Source: CAD feature listing. Evaluate the final solid. Frame: model axes, mm. Face numbers are marked on the shaded views. A direction names the side the tool comes from. Give positions to 0.01 mm unless a question says otherwise; leave off trailing zeros. Write each loop counter-clockwise with the first axis right and the second up, starting at its lowest first coordinate (ties: lowest second). Pieces come first, ordered by that corner, then holes.
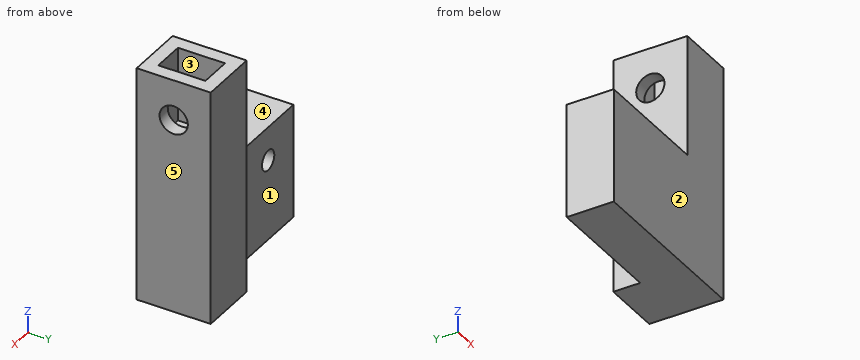
```python
from build123d import *

# Parameters (mm, degrees)
SKETCH_1_W          = 8.8
SKETCH_1_H          = 11
EXTRUDE_1_DEPTH     = 35
SKETCH_2_W          = 4.8
SKETCH_2_H          = 7
CUT_EXTRUDE_1_DEPTH = 11
SKETCH_3_R          = 2.1
CUT_EXTRUDE_2_DEPTH = 11
SKETCH_4_W          = 17
SKETCH_4_H          = 7
EXTRUDE_2_DEPTH     = 18
SKETCH_5_R          = 1.5
CUT_EXTRUDE_3_DEPTH = 4.5


with BuildPart() as part:
    # 草图1 → 凸台-拉伸1 (new body)
    with BuildSketch(Plane.XY):
        Rectangle(SKETCH_1_W, SKETCH_1_H)
    extrude(amount=-EXTRUDE_1_DEPTH)

    # 草图2 → 切除-拉伸1 (cut)
    with BuildSketch(Plane.XY):
        Rectangle(SKETCH_2_W, SKETCH_2_H)
    extrude(amount=-CUT_EXTRUDE_1_DEPTH, mode=Mode.SUBTRACT)

    # 草图3 → 切除-拉伸2 (cut)
    with BuildSketch(Plane.ZY.offset(4.4)):
        with Locations((-6, 0)):
            Circle(SKETCH_3_R)
    extrude(amount=-CUT_EXTRUDE_2_DEPTH, mode=Mode.SUBTRACT)

    # 草图4 → 凸台-拉伸2 (add)
    with BuildSketch(Plane.ZY.offset(4.4)):
        with Locations((-26.5, -2)):
            Rectangle(SKETCH_4_W, SKETCH_4_H)
    extrude(amount=EXTRUDE_2_DEPTH)

    # 草图5 → 切除-拉伸3 (cut)
    with BuildSketch(Plane(origin=(0, 1.5, 0), x_dir=(1, 0, 0), z_dir=(0, 1, 0))):
        with Locations((-16.24, 23)):
            Circle(SKETCH_5_R)
    extrude(amount=-CUT_EXTRUDE_3_DEPTH, mode=Mode.SUBTRACT)


solid = part.part
```
1. Cut plane C-C, the plane y = -2.5. Return the cut outline in (x, z), then the cut area to 3 significant figures.
2. Contact query for flat-ended pins moving along their axis: P1, Ø5.5, axis at x = -9, y = -2, coming from the +Z side; P2, Ø4, axis at y = 0, z = -6, coming from the -X side; P3, Ø1.4, axis at x = 0.5, y = 0, coming from the +Z side; P4, Ø5, axis at y = 0, z = -6, coming from the -X side. Output: stop coordinate, or through.
3. Cut plane B-B, the plane z = -6. Return the cut outline in (x, y).
4. Cut plane D-D, the plane x = -16.24. Return the cut outline in (y, z).
5. Access query for the marked faces 1 and 2. Directions: +Z, -Z, +X, -X, +Y, -Y. A direction counts if a zero-diameter tool reaches every point of the face in a straight line with its end or side. Return the directions, or none.
6. Mould query, pull axis X, two halves, no side actions, for the marked faces 3, 4 and 5. Classes: +X half, -X half, draft (parallel to the pull), parting line (faces both ways), or undercut.
7. Cut plane A-A, the plane y = 0. Return the cut outline in (x, z).
8. Line query: L1, parallel to Y at x = 3.8, z = -6; L2, parallel to Z at x = -16.24, y = 0.25; L3, parallel to X at y = 2.75, z = -6. Output: solid intervals per line, ascending.
Response values:
1. outline: (-22.4, -35) - (4.4, -35) - (4.4, 0) - (2.4, 0) - (2.4, -11) - (-2.4, -11) - (-2.4, 0) - (-4.4, 0) - (-4.4, -18) - (-22.4, -18) - close; hole circle Ø3 at (-16.24, -23)
1. area: 554 mm2
2. P1: stops at z = -18
2. P2: passes through
2. P3: stops at z = -11
2. P4: stops at x = -4.4
3. outline: (-4.4, -5.5) - (4.4, -5.5) - (4.4, -2.1) - (2.4, -2.1) - (2.4, -3.5) - (-2.4, -3.5) - (-2.4, -2.1) - (-4.4, -2.1) - close; (-4.4, 2.1) - (-2.4, 2.1) - (-2.4, 3.5) - (2.4, 3.5) - (2.4, 2.1) - (4.4, 2.1) - (4.4, 5.5) - (-4.4, 5.5) - close
4. outline: (-5.5, -35) - (1.5, -35) - (1.5, -24.5) - (-3, -24.5) - (-3, -21.5) - (1.5, -21.5) - (1.5, -18) - (-5.5, -18) - close
5. face 1: +Z, -Z, -X, +Y
5. face 2: +Z, -Z, +X, -X, -Y
6. face 3: undercut
6. face 4: draft
6. face 5: +X half
7. outline: (-22.4, -35) - (4.4, -35) - (4.4, -8.1) - (2.4, -8.1) - (2.4, -11) - (-2.4, -11) - (-2.4, -8.1) - (-4.4, -8.1) - (-4.4, -18) - (-22.4, -18) - close; (-4.4, -3.9) - (-2.4, -3.9) - (-2.4, 0) - (-4.4, 0) - close; (2.4, -3.9) - (4.4, -3.9) - (4.4, 0) - (2.4, 0) - close; hole circle Ø3 at (-16.24, -23)
8. L1: y = -5.5 to -2.1, 2.1 to 5.5
8. L2: z = -35 to -24.5, -21.5 to -18
8. L3: x = -4.4 to -2.4, 2.4 to 4.4
